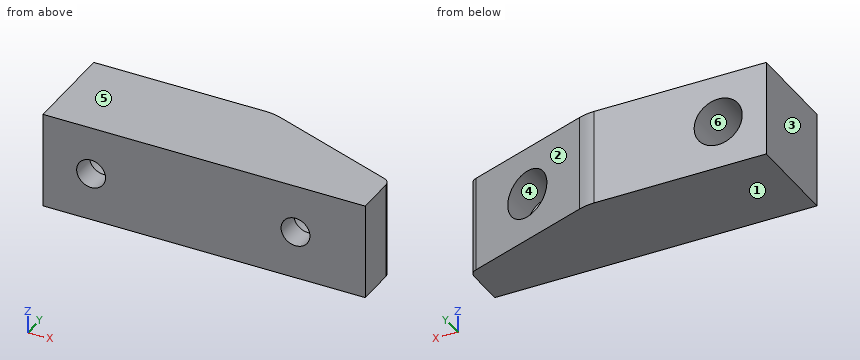
from build123d import *

# Parameters (mm, degrees)
SKETCH1_W               = 75
SKETCH1_H               = 40
SKETCH1_R               = 10
BOSS_EXTRUDE1_DEPTH     = 40
SKETCH1_4_W             = 59
SKETCH1_4_H             = 40
SKETCH1_4_R             = 10
BOSS_EXTRUDE2_DEPTH     = 40
CUT_EXTRUDE2_DEPTH      = 146.451022685
CUT_EXTRUDE2_DEPTH_BACK = 40
FILLET2_R               = 20
FILLET3_R               = 4
SKETCH1_5_R             = 10
SKETCH1_5_R_2           = 6
BOSS_EXTRUDE3_DEPTH     = 10


with BuildPart() as part:
    # Sketch1 → Boss-Extrude1 (new body)
    with BuildSketch(Plane(origin=(0, 0, 0), x_dir=(1, 0, 0), z_dir=(0, 1, 0))):
        with Locations((37.5, 20)):
            Rectangle(SKETCH1_W, SKETCH1_H)
        with Locations(Location((20, 20, 0), (0, 0, 270))):
            Circle(SKETCH1_R, mode=Mode.SUBTRACT)
    extrude(amount=BOSS_EXTRUDE1_DEPTH)

    # Sketch1_4 → Boss-Extrude2 (add)
    with BuildSketch(Plane(origin=(0, 0, 0), x_dir=(1, 0, 0), z_dir=(0, 1, 0))):
        with Locations((104.5, 20)):
            Rectangle(SKETCH1_4_W, SKETCH1_4_H)
        with Locations(Location((105, 20, 0), (0, 0, 270))):
            Circle(SKETCH1_4_R, mode=Mode.SUBTRACT)
    extrude(amount=BOSS_EXTRUDE2_DEPTH)

    # Sketch5 → Cut-Extrude2 (cut, two sides: drawn at the far end of the back side and taken through both)
    with BuildSketch(Plane(origin=(0, 0, -40), x_dir=(-1, 0, 0), z_dir=(0, 0, -1)).offset(-CUT_EXTRUDE2_DEPTH_BACK)):
        Polygon((-398.986226701, -75.317131538), (-134, 19), (-75, 40), (189.986226701, 134.317131538), (1.351963626, 664.289584939), (-587.620489776, 454.655321864), align=None)
    extrude(amount=CUT_EXTRUDE2_DEPTH + CUT_EXTRUDE2_DEPTH_BACK, mode=Mode.SUBTRACT)

    # Fillet2
    fillet2_edges = [part.edges().sort_by_distance(p)[0] for p in [
        (75, 40, -20),
    ]]
    fillet(fillet2_edges, radius=FILLET2_R)

    # Fillet3
    fillet3_edges = [part.edges().sort_by_distance(p)[0] for p in [
        (134, 19, -20),
    ]]
    fillet(fillet3_edges, radius=FILLET3_R)

    # Sketch1_5 → Boss-Extrude3 (add)
    # profile 1 of 2: a face of its own
    with BuildSketch(Plane(origin=(0, 0, 0), x_dir=(1, 0, 0), z_dir=(0, 1, 0))):
        with Locations(Location((20, 20, 0), (0, 0, 270))):
            Circle(SKETCH1_5_R)
        with Locations(Location((20, 20, 0), (0, 0, 270))):
            Circle(SKETCH1_5_R_2, mode=Mode.SUBTRACT)
    # profile 2 of 2: a face of its own
    with BuildSketch(Plane(origin=(0, 0, 0), x_dir=(1, 0, 0), z_dir=(0, 1, 0))):
        with Locations((105, 20)):
            Circle(SKETCH1_5_R)
        with Locations(Location((105, 20, 0), (0, 0, 270))):
            Circle(SKETCH1_5_R_2, mode=Mode.SUBTRACT)
    extrude(amount=BOSS_EXTRUDE3_DEPTH)


solid = part.part
Can you work these out from the model? Positions are in its coordinate system, mm. Face numbers are marked on the shaded views. A direction names the side the tool comes from. Coordinates: 2 decimals unless noted, no trailing zeros. Order: outer loops, then holes, each group sorted by start corner. A loop starts at its lowest first (then second) coordinate and runs counter-clockwise, first axis right, second up. Notation, with made-up numbers: (-22.5, 86.5) -> (12.5, 86.5) arc R6 cw to (12.5, 97.5) -> close; hole circle Ø2 at (-8, 84.5). An arc over 180 degrees is marked (long way). Use one line per item in the form item = value.
Q1. Imagine slicing it at D-D, the plane y = 26.5. List the corners of the cut face in (x, z) for me.
From the geometry:
outline = (0, -40) -> (112.93, -40) -> (112.93, -26.09) arc R10 cw (long way) to (112.93, -13.91) -> (112.93, 0) -> (0, 0) -> close; hole circle Ø20 at (20, -20)
Q2. Imagine slicing it at C-C, the plane z = -7. List the corners of the cut face in (x, y) for me.
From the geometry:
outline = (0, 0) -> (134, 0) -> (134, 16.18) arc R4 ccw to (131.34, 19.95) -> (78.25, 38.84) arc R20 ccw to (71.55, 40) -> (0, 40) -> close
Q3. Imagine slicing it at B-B, the plane y = 6.5. List the corners of the cut face in (x, z) for me, then the cut area to 3 significant figures.
From the geometry:
outline = (0, -40) -> (134, -40) -> (134, 0) -> (0, 0) -> close; hole circle Ø12 at (20, -20); hole circle Ø12 at (105, -20)
area = 5,130 mm²
Q4. Will these pins go through, and if not, where does the flat tip stop? P1, Ø7, axis at x = 105, z = -20, coming from the -Y side; P2, Ø6, axis at x = 25, z = -18, coming from the +Y side.
From the geometry:
P1 = through
P2 = 10
Q5. I need wall thicknesses on L1, parallel to X at y = 26, z = -20; L2, parallel to X at y = 5, z = -20; L3, parallel to Z at x = 105, y = 21.5. Which ranges of each line are inside material? Lowest first, please.
From the geometry:
L1 = 0 to 10, 30 to 95
L2 = 0 to 14, 26 to 99, 111 to 134
L3 = -40 to -30, -10 to 0
Q6. We'd pull the mould along X, two halves only. Please class the marked faces 1, 2, 3 and 4: released by +X, released by -X, zero draft, split by the parting line, or undercut.
From the geometry:
face_1 = zero draft
face_2 = released by +X
face_3 = released by -X
face_4 = undercut
Q7. Which directions (+Z, -Z, +X, -X, +Y, -Y) give clear straight access to the entire face, cutting with the end or side of a thin tool? Please do the marked faces 5 and 6.
From the geometry:
face_5 = +Z, +X, -X, +Y, -Y
face_6 = +Y
Q8. Imagine slicing it at A-A, the plane x = 20. List the corners of the cut face in (y, z) for me.
From the geometry:
outline = (0, -40) -> (40, -40) -> (40, -30) -> (10, -30) -> (10, -26) -> (0, -26) -> close; (0, -14) -> (10, -14) -> (10, -10) -> (40, -10) -> (40, 0) -> (0, 0) -> close
